Source: three-view drawing plus pictorial views. Frame: mm from the lowest corner of the part. A direction names the side the tool comes from. Give positions to 0.01 mm unless a question says otherwise; leave off trailing zeros. Loops run counter-clockwise (first coordinate to the right, second up) from the corner with the lowest first, then second, coordinate; pieces in that order, holes last. Notation, with made-up numbers: M 20.25,82 L 71.25,82 A24 cw 71.25,119 Z; hole C 29,45 d3. An arc over 180 degrees is marked long. Write item = value, one per line.
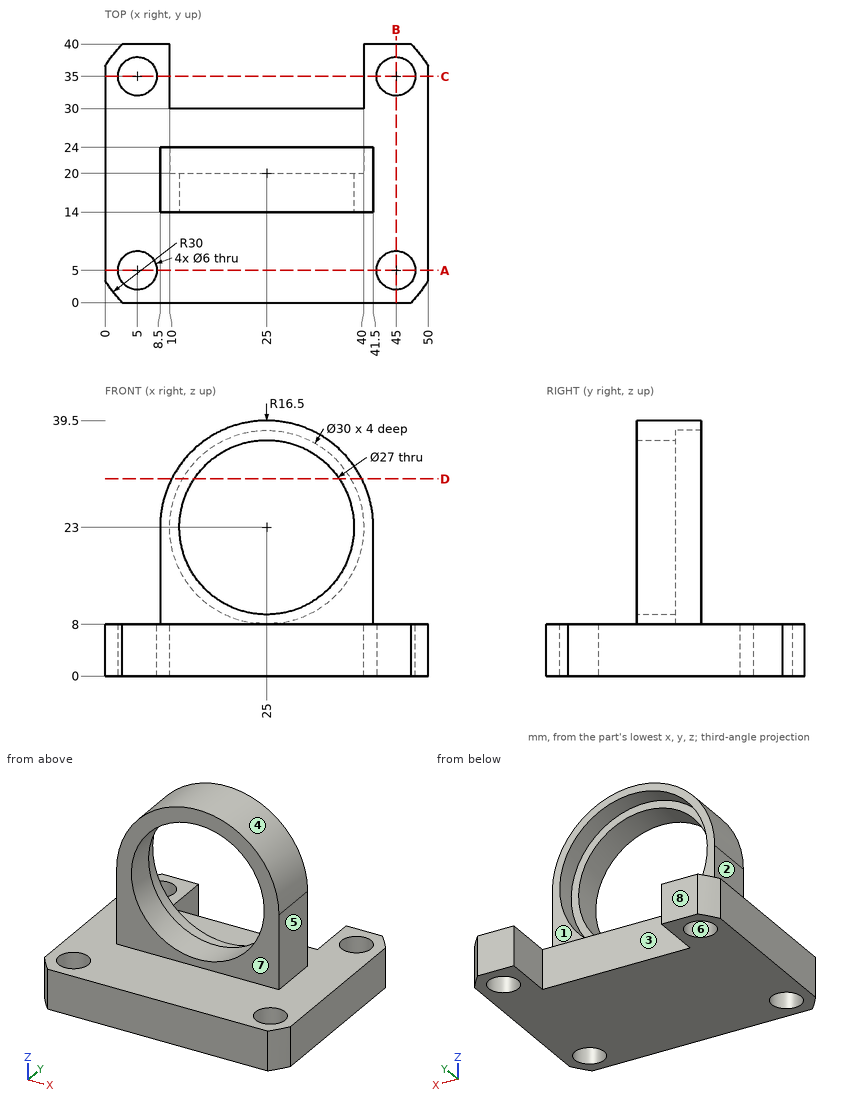
1. Cut plane D-D, the plane z = 30.5. Return the cut outline in (x, y).
Derived:
outline = M 10.3,14 L 13.78,14 L 13.78,20 L 12.01,20 L 12.01,24 L 10.3,24 Z; M 36.22,14 L 39.7,14 L 39.7,24 L 37.99,24 L 37.99,20 L 36.22,20 Z
2. First-contact query: pin 1 Ø5 at (x, y) = (5, 5) entering from -Z; pin 2 Ø2 at (y, z) = (23, 22.5) entering from +X; pin 3 Ø6.5 at (x, z) = (23.5, 5.5) entering from +Y; pin 4 Ø6 at (x, z) = (37.5, 13) entering from +Y. Flat tips, straight axial feed; report the tip coordinate or a pass-through.
Derived:
pin_1 = through
pin_2 = 41.5
pin_3 = 30
pin_4 = 24
3. Cut plane C-C, the plane y = 35. Return the cut outline in (x, z).
Derived:
outline = M 0,0 L 2,0 L 2,8 L 0,8 Z; M 8,0 L 10,0 L 10,8 L 8,8 Z; M 40,0 L 42,0 L 42,8 L 40,8 Z; M 48,0 L 50,0 L 50,8 L 48,8 Z
4. Reachability of the marked faces 1, 2, 3, 4 and 5 from +Z, -Z, +X, -X, +Y, -Y: full face, straight path, thin tool, end or side. Return the list, or none.
Derived:
face_1 = +Z, +X, -X, +Y
face_2 = +Z, -X, +Y, -Y
face_3 = +Z, -Z, +Y
face_4 = +Z, +Y, -Y
face_5 = +Z, +X, +Y, -Y
5. Material intervals for probe 1 along Y at (x, z) = (5, 4); probe 2 along X at (y, z) = (22, 23); probe 3 along Z at (x, y) = (47.5, 21), sorted ascending. Write a range as from..to.
Derived:
probe_1 = 0..2, 8..32, 38..40
probe_2 = 8.5..10, 40..41.5
probe_3 = 0..8
6. Pull-direction query (Y, two-part tool) for the marked faces 6, 7 and 8; classes: +Y half, -Y half, draft (parallel to the pull), parting line (faces both ways), or undercut.
Derived:
face_6 = undercut
face_7 = -Y half
face_8 = +Y half
7. Cut plane A-A, the plane y = 5. Return the cut outline in (x, z), then the cut area to 3 significant figures.
Derived:
outline = M 0,0 L 2,0 L 2,8 L 0,8 Z; M 8,0 L 42,0 L 42,8 L 8,8 Z; M 48,0 L 50,0 L 50,8 L 48,8 Z
area = 304 mm²
8. Cut plane B-B, the plane x = 45. Return the cut outline in (y, z).
Derived:
outline = M 0,0 L 2,0 L 2,8 L 0,8 Z; M 8,0 L 32,0 L 32,8 L 8,8 Z; M 38,0 L 40,0 L 40,8 L 38,8 Z
